```python
from build123d import *

# Parameters (mm, degrees)
PAD_DEPTH       = 9
POCKET_DEPTH    = 6
SKETCH002_W     = 26.5
SKETCH002_H     = 35
POCKET001_DEPTH = 6
SKETCH003_W     = 192.75
SKETCH003_H     = 5.95
PAD001_DEPTH    = 3
SKETCH004_R     = 0.85
POCKET002_DEPTH = 553.365942
SKETCH005_W     = 26.5
SKETCH005_H     = 7.75
PAD002_DEPTH    = 3


with BuildPart() as part:
    # Sketch → Pad (new body)
    with BuildSketch(Plane.XY):
        with BuildLine():
            ThreePointArc((-82.5, 45), (-127.5, 0), (-82.5, -45))
            Line((-82.5, -45), (82.5, -45))
            ThreePointArc((82.5, -45), (127.5, 0), (82.5, 45))
            Line((-82.5, 45), (82.5, 45))
        make_face()
    extrude(amount=PAD_DEPTH)

    # Sketch001 (on Face6 of Pad) → Pocket (cut)
    with BuildSketch(Plane.XY.offset(9)):
        with BuildLine():
            ThreePointArc((-97.5, 6), (-103.5, 0), (-97.5, -6))
            Line((-97.5, -6), (97.5, -6))
            ThreePointArc((97.5, -6), (103.5, 0), (97.5, 6))
            Line((-97.5, 6), (97.5, 6))
        make_face()
    extrude(amount=-POCKET_DEPTH, mode=Mode.SUBTRACT)

    # Sketch002 (on Face5 of Pocket) → Pocket001 (cut)
    with BuildSketch(Plane.XY.offset(9)):
        with Locations((0, -27.5)):
            Rectangle(SKETCH002_W, SKETCH002_H)
    extrude(amount=-POCKET001_DEPTH, mode=Mode.SUBTRACT)

    # Sketch003 (on Face5 of Pocket001) → Pad001 (join)
    with BuildSketch(Plane.XY.offset(9)):
        with BuildLine():
            ThreePointArc((-82.5, 45), (-127.5, 0), (-82.5, -45))
            Line((-82.5, -45), (82.5, -45))
            ThreePointArc((82.5, -45), (127.5, 0), (82.5, 45))
            Line((-82.5, 45), (82.5, 45))
        make_face()
        Rectangle(SKETCH003_W, SKETCH003_H, mode=Mode.SUBTRACT)
    extrude(amount=PAD001_DEPTH)

    # Sketch004 (on Face12 of Pad001) → Pocket002 (cut, through all)
    with BuildSketch(Plane.XY.offset(12)):
        with Locations((-80, -8)):
            Circle(SKETCH004_R)
        with Locations((-63, -8)):
            Circle(SKETCH004_R)
        with Locations((-63, 8)):
            Circle(SKETCH004_R)
        with Locations((-80, 8)):
            Circle(SKETCH004_R)
    pocket002 = extrude(amount=-POCKET002_DEPTH, mode=Mode.SUBTRACT)

    # Sketch005 (on Face10 of Pocket002) → Pad002 (join)
    with BuildSketch(Plane.XY.offset(3)):
        with Locations((0, -37.125)):
            Rectangle(SKETCH005_W, SKETCH005_H)
    extrude(amount=PAD002_DEPTH)

    # Mirrored: Pocket002 across Sketch004 V_Axis
    add(pocket002.mirror(Plane(origin=(0, 0, 12), x_dir=(0, 0, 1), z_dir=(1, 0, 0))), mode=Mode.SUBTRACT)


solid = part.part
```
Here's how the part is built. I have some questions about the finished solid (model axes, mm). A direction names the side the tool comes from. Coordinates: 2 decimals unless noted, no trailing zeros. Loops run counter-clockwise (first coordinate to the right, second up) from the corner with the lowest first, then second, coordinate; pieces in that order, holes last. Notation, with made-up numbers: (23.5, 81.5) - (35.5, 81.5) arc R15 ccw to (35.5, 96.5) - close; hole circle Ø8 at (66.5, 27.25). An arc over 180 degrees is marked (long way). Return JSON: item names as keys, results as strings. Group by question number.
Item 1: On a 3-axis mill with a long thin cutter (end or side, diameter ignored), from which of +Z, -Z, +X, -X, +Y, -Y can I reach the whole of each face in a straight line? I mean faces 1 (the face through (127.49, -0.99, 5.92)), 2 (the face through (0, -10, 6)), 3 (the face through (0, -37, 6)). Say none if no direction works.
Item 2: We'd pull the mould along Z, two halves only. Please class faces 4 (the face through (0, -21, 3)), 5 (the face through (-1, 45, 6)), 6 (the face through (-2, 11, 12)): +Z half, -Z half, draft (parallel to the pull), parting line (faces both ways), or undercut.
Item 3: If we section it at B-B on x = 23: Write out the boundary of the cut face in (y, z) (3 decimals).
Item 4: If we section it at A-A on y = -36: Write out the boundary of the cut face in (x, z).
Item 5: Will these pins go through, and if not, where does the flat tip stop? P1, Ø2, axis at y = 16, z = 5.5, coming from the +X side; P2, Ø1, axis at x = 63, y = 8, coming from the -Z side; P3, Ø1.5, axis at x = -86.5, z = 5, coming from the +Y side; P4, Ø2.5, axis at x = -1.5, z = 5, coming from the -Y side.
Item 6: I need wall thicknesses on line 1 (Y direction, x = -63, z = 6); line 2 (Y direction, x = 64.5, z = 11) (3 decimals); line 3 (Z direction, x = -8, y = -37). Which ranges of each line are inside material? Lowest first, please. Write a range as from..to.
Item 7: If we section it at C-C on y = 37: Write out the boundary of the cut face in (x, z), and give its area (3 significant figures).
Calculated:
{
 "1": {"face 1": "+Z, -Z, +X", "face 2": "none", "face 3": "-Y"},
 "2": {"face 4": "undercut", "face 5": "draft", "face 6": "+Z half"},
 "3": {"outline": "(-45, 0) - (45, 0) - (45, 12) - (2.975, 12) - (2.975, 9) - (6, 9) - (6, 3) - (-6, 3) - (-6, 9) - (-2.975, 9) - (-2.975, 12) - (-45, 12) - close"},
 "4": {"outline": "(-109.5, 0) - (109.5, 0) - (109.5, 12) - (-109.5, 12) - close; hole (-13.25, 6) - (13.25, 6) - (13.25, 9) - (-13.25, 9) - close"},
 "5": {"P1": "stops at x = 124.93", "P2": "passes through", "P3": "stops at y = 44.88", "P4": "stops at y = -41"},
 "6": {"line 1": "y = -45..-8.85, -7.15..-6, 6..7.15, 8.85..45", "line 2": "y = -45..-2.975, 2.975..45", "line 3": "z = 0..6, 9..12"},
 "7": {"outline": "(-108.11, 0) - (108.11, 0) - (108.11, 12) - (-108.11, 12) - close", "area": "2,590 mm^2"}
}
